Can you work these out from the model? Positions are in its coordinate system, mm. Face numbers are marked on the shaded views. Round coordinates to 2 decimals unless told otherwise and drop trailing zeros. Order: outer loops, then holes, each group sorted by start corner. A loop starts at its lowest first (then second) coordinate and runs counter-clockwise, first axis right, second up.
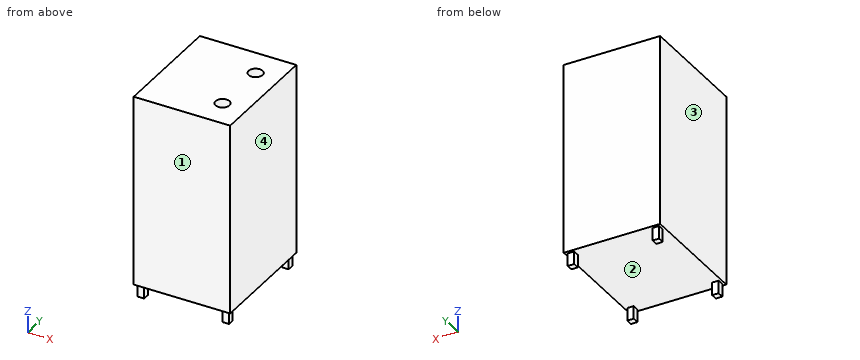
from build123d import *

# Parameters (mm, degrees)
F0_W     = 750
F0_H     = 900
F1_DEPTH = 1490
F2_W     = 50
F2_H     = 50
F3_DEPTH = 100
F4_R     = 55
F5_DEPTH = 200


with BuildPart() as f1:
    # F0 (on Top) → F1 (new body)
    with BuildSketch(Plane.XY):
        Rectangle(F0_W, F0_H)
    extrude(amount=-F1_DEPTH)

    # F2 (on face) → F3 (join)
    with BuildSketch(Plane(origin=(0, 0, -1490), x_dir=(1, 0, 0), z_dir=(0, 0, -1))):
        with Locations((-330, 405)):
            Rectangle(F2_W, F2_H)
        with Locations((330, 405)):
            Rectangle(F2_W, F2_H)
        with Locations((-330, -405)):
            Rectangle(F2_W, F2_H)
        with Locations((330, -405)):
            Rectangle(F2_W, F2_H)
    extrude(amount=F3_DEPTH)

    # F4 (on face) → F5 (cut)
    with BuildSketch(Plane.XY):
        with Locations((187.5, 225)):
            Circle(F4_R)
        with Locations((187.5, -225)):
            Circle(F4_R)
    extrude(amount=-F5_DEPTH, mode=Mode.SUBTRACT)


solid = f1.part
(1) I want a section at C-C, the plane x = -18.5. List the corners of the cut face in (y, z) for me, plus the area to 3 significant figures.
(2) I want a section at A-A, the plane y = -225. List the corners of the cut face in (x, z) for me.
(3) I'm going to push flat-ended pins straight in: pin 1 Ø25 at (y, z) = (-408, -1562.5) entering from +X; pin 2 Ø15 at (x, z) = (338.5, -1563.5) entering from -Y; pin 3 Ø1 at (x, y) = (-59.5, 182.5) entering from +Z; pin 4 Ø6 at (x, y) = (185.5, 77.5) entering from -Z. Where does each tip first touch, or does it pass through?
(4) Please list where these lines run through material, in increasing order: probe 1 along Y at (x, z) = (187.5, -43); probe 2 along Z at (x, y) = (-83, 124.5); probe 3 along Z at (x, y) = (191, -174).
(5) I want a section at D-D, the plane y = 191. List the corners of the cut face in (x, z) for me, plus the area to 3 significant figures.
(6) I want a section at B-B, the plane x = 187.5. List the corners of the cut face in (y, z) for me.
(7) If we mould it in two halves opening along X, with no side actions, what happens to the marked faces 1, 2, 3 and 4? For each: pulls with the +X half, pulls with the -X half, needs draft (parallel to the pull), parting line crosses it, or undercut.
Ans:
1. outline: (-450, -1490) - (450, -1490) - (450, 0) - (-450, 0) - close
1. area: 1,340,000 mm2
2. outline: (-375, -1490) - (375, -1490) - (375, 0) - (242.5, 0) - (242.5, -200) - (132.5, -200) - (132.5, 0) - (-375, 0) - close
3. pin 1: stops at x = 355
3. pin 2: stops at y = -430
3. pin 3: stops at z = 0
3. pin 4: stops at z = -1490
4. probe 1: y = -450 to -280, -170 to 170, 280 to 450
4. probe 2: z = -1490 to 0
4. probe 3: z = -1490 to -200
5. outline: (-375, -1490) - (375, -1490) - (375, 0) - (230.73, 0) - (230.73, -200) - (144.27, -200) - (144.27, 0) - (-375, 0) - close
5. area: 1,100,000 mm2
6. outline: (-450, -1490) - (450, -1490) - (450, 0) - (280, 0) - (280, -200) - (170, -200) - (170, 0) - (-170, 0) - (-170, -200) - (-280, -200) - (-280, 0) - (-450, 0) - close
7. face 1: needs draft
7. face 2: undercut
7. face 3: pulls with the -X half
7. face 4: pulls with the +X half
